Input: dimensioned drawing with shaded views. Units: mm. Origin: part minimum x, y, z. Round coordinates to 2 decimals unless told otherwise and drop trailing zeros. Order: outer loops, then holes, each group sorted by start corner. A loop starts at its lowest first (then second) coordinate and runs counter-clockwise, first axis right, second up. Notation, with made-up numbers: (1.5, 43.25) - (53.5, 43.25) arc R21 cw to (53.5, 78.25) - close; hole circle Ø8 at (7, 22.25). An arc over 180 degrees is marked (long way). Return JSON: item names as keys, results as strings. Group by question number.
1) Section C-C, the plane y = 2.65. Return loops of the section in (x, z) (3 decimals).
2) Section B-B, the plane z = 5. Return loops of the section in (x, y) (3 decimals), plus the area to 3 significant figures.
3) Ray query, line 1 (X direction, y = 1.85, z = 10) (3 decimals); line 2 (X direction, y = 2.35, z = 5); line 3 (Z direction, x = 11.5, y = 2.25). Return the intervals inside material, ascending. Write a range as from..to.
4) Contact query for flat-ended pins moving along their axis: P1, Ø12, axis at x = 17.5, z = 6, coming from the +Y side (3 decimals); P2, Ø2, axis at x = 17.35, z = 5, coming from the +Y side. Output: stop coordinate, or through.
5) Section A-A, the plane x = 17.35. Return loops of the section in (y, z) (3 decimals), plus the area to 3 significant figures.
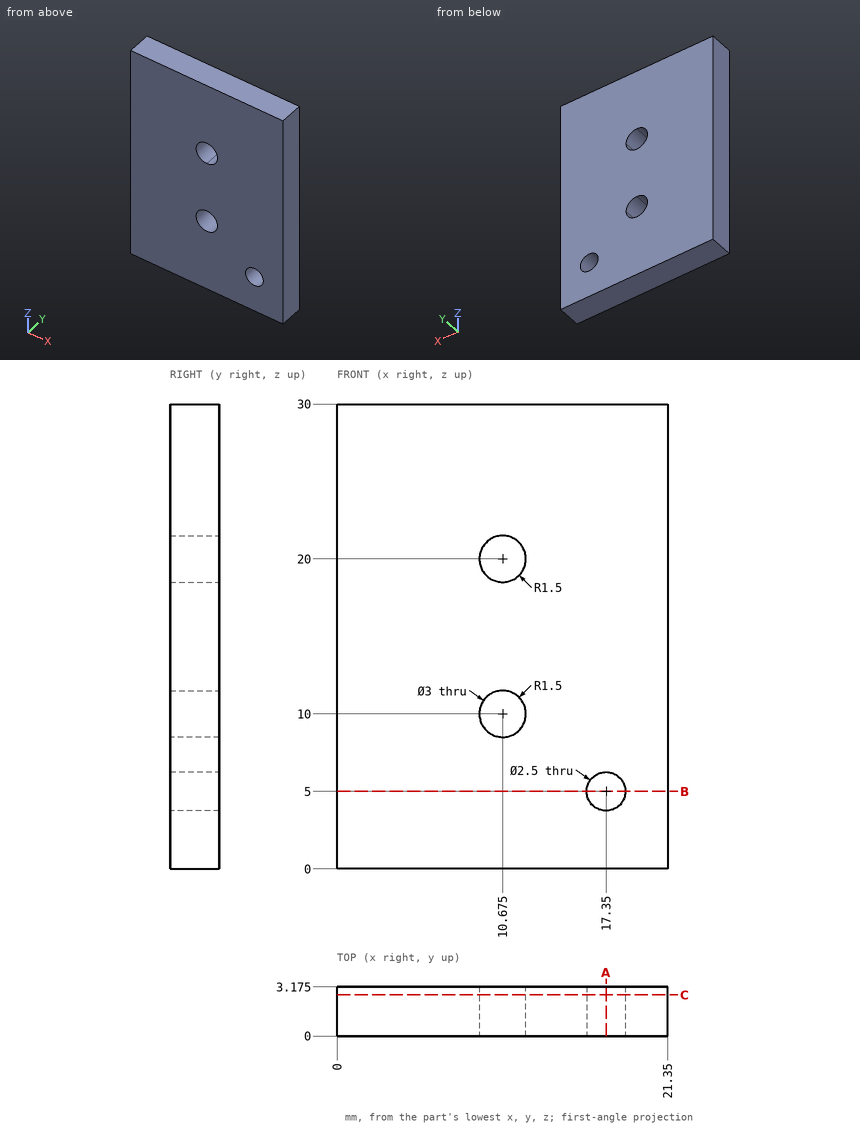
Geometry check:
{
 "1": {"outline": "(0, 0) - (21.35, 0) - (21.35, 30) - (0, 30) - close; hole circle Ø3 at (10.675, 10); hole circle Ø3 at (10.675, 20); hole circle Ø2.5 at (17.35, 5)"},
 "2": {"outline": "(0, 0) - (16.1, 0) - (16.1, 3.175) - (0, 3.175) - close; (18.6, 0) - (21.35, 0) - (21.35, 3.175) - (18.6, 3.175) - close", "area": "59.8 mm2"},
 "3": {"line 1": "0..9.175, 12.175..21.35", "line 2": "0..16.1, 18.6..21.35", "line 3": "0..8.75, 11.25..18.75, 21.25..30"},
 "4": {"P1": "y = 3.175", "P2": "through"},
 "5": {"outline": "(0, 0) - (3.175, 0) - (3.175, 3.75) - (0, 3.75) - close; (0, 6.25) - (3.175, 6.25) - (3.175, 30) - (0, 30) - close", "area": "87.3 mm2"}
}
